Could you check a few things on this model? Use its own coordinates, in mm. A direction names the side the tool comes from. Give positions to 0.01 mm unless a question says otherwise; leave off trailing zeros. Write each loop counter-clockwise with the first axis right and the second up, starting at its lowest first coordinate (ties: lowest second). Pieces come first, ordered by that corner, then holes. Notation, with made-up numbers: (27.25, -21) -> (31.25, -21) arc R21 ccw to (31.25, 16) -> close; hole circle Ø10 at (-18, 85.5). An arc over 180 degrees is marked (long way). Write item = value, one per line. Start each with the question number.
Autodesk Inventor part; units mm, degrees
ref_plane "L_XY" through (12.2, 0, 0) normal (1, 0, 0) x (0, 0, -1)
ref_plane "L_YZ" through (12.2, 0, 0) normal (0, 0, -1) x (0, 1, 0)
ref_plane "L_ZX" through (12.2, 0, 0) normal (0, 1, 0) x (1, 0, 0)
sketch "Sketch_1" plane through (0, 0, 0) normal (0, 0, 1) x (1, 0, 0)
  line L0 (11.9, 0) -> (0, 0)
  line L1 (0, 0) -> (0, 8.2)
  line L2 (0, 8.2) -> (0.2, 8.4)
  line L3 (0.2, 8.4) -> (11.9, 8.4)
  line L4 (11.9, 8.4) -> (11.9, 0)
  line L5 (11.9, 0) -> (0, 0)
revolve "Revolution1" add sketch "Sketch_1" angle 360 about axis through (11.9, 0, 0) along (1, 0, 0)
sketch "Sketch_6" plane through (0, 0, 0) normal (1, 0, 0) x (0, 1, 0)
  line L0 (0, 0.6) -> (-8.4, 0.6)
  line L1 (-8.4, 0.6) -> (-8.4, -0.6)
  line L2 (-8.4, -0.6) -> (0, -0.6)
  line L3 (0, -0.6) -> (0, 0.6)
extrude "Extrusion1" cut sketch "Sketch_6" along normal blind 9
sketch "Sketch_7" plane through (4, 0, 0) normal (1, 0, 0) x (0, 0, -1)
  line L0 (-8.4, -5) -> (8.4, -5)
  line L1 (8.4, -5) -> (8.4, -7.75)
  line L2 (8.4, -7.75) -> (3, -7.75)
  line L3 (3, -7.75) -> (3, -6.5)
  line L4 (3, -6.5) -> (0.6, -6.5)
  line L5 (0.6, -6.5) -> (0.6, -5)
  line L6 (0.6, -5) -> (8.4, -5)
revolve "Revolution2" cut sketch "Sketch_7" angle 360 about axis through (4, -5, 8.4) along (0, 0, 1)
sketch "Sketch_13" plane through (4, 0, 0) normal (1, 0, 0) x (0, 0, -1)
  line L0 (-8.4, -5) -> (8.4, -5)
  line L1 (-0.6, -5) -> (-0.6, -6.2295)
  line L2 (-0.6, -6.2295) -> (-8.4, -6.2295)
  line L3 (-8.4, -6.2295) -> (-8.4, -5)
  line L4 (-8.4, -5) -> (-0.6, -5)
revolve "Revolution3" cut sketch "Sketch_13" angle 360 about axis through (4, -5, 8.4) along (0, 0, 1)
thread "Thread1"
sketch "Sketch_2" plane through (11.9, 0, 0) normal (1, 0, 0) x (0, 0, -1)
  line L0 (-9.4, 8.9) -> (-9.4, -8.9)
  line L1 (-9.4, -8.9) -> (9.4, -8.9)
  line L2 (9.4, -8.9) -> (9.4, 8.9)
  line L3 (9.4, 8.9) -> (-9.4, 8.9)
  line L4 (-8.4, 2.3) -> (-8.4, -2.3)
  line L5 (-8.4, -2.3) -> (8.4, -2.3)
  line L6 (8.4, -2.3) -> (8.4, 2.3)
  line L7 (8.4, 2.3) -> (-8.4, 2.3)
extrude "Extrusion2" cut sketch "Sketch_2" against normal blind 2.9
sketch "Sketch_3" plane through (0, 0, 0) normal (0, 0, 1) x (1, 0, 0)
  line L0 (11.9, 0) -> (0, 0)
  line L1 (0, 0) -> (0, 3)
  line L2 (0, 3) -> (11.9, 3)
  line L3 (11.9, 3) -> (11.9, 0)
  line L4 (11.9, 0) -> (0, 0)
revolve "Revolution4" cut sketch "Sketch_3" angle 360 about axis through (11.9, 0, 0) along (1, 0, 0)
sketch "Sketch_17" plane through (0, 0, 0) normal (1, 0, 0) x (0, 0, -1)
  line L0 (-0.6, 0) -> (0.6, 0)
  line L1 (0.6, 0) -> (0.6, 4.44)
  line L2 (0.6, 4.44) -> (-0.6, 4.44)
  line L3 (-0.6, 4.44) -> (-0.6, 0)
extrude "Extrusion3" cut sketch "Sketch_17" along normal blind 11.9
ref_plane "L_XY" through (12.2, 0, 0) normal (1, 0, 0) x (0, 0, -1)
ref_plane "L_YZ" through (12.2, 0, 0) normal (0, 0, -1) x (0, 1, 0)
ref_plane "L_ZX" through (12.2, 0, 0) normal (0, 1, 0) x (1, 0, 0)
ref_plane "screw_XY" through (4, -5, -3) normal (0, 0, -1) x (1, 0, 0)
ref_plane "screw_YZ" through (4, -5, -3) normal (1, 0, 0) x (0, -1, 0)
ref_plane "screw_ZX" through (4, -5, -3) normal (0, -1, 0) x (0, 0, -1)
properties part number "MCOC17-6_c"
(1) Imagine slicing it at C-C (x = 8.75). Please give me the cut outline in (y, z), then the cut area to 3 significant figures.
(2) We'd pull the mould along Z, two halves only. Please class faces 1 (the cylindrical face through (6, 0, 3)), 2 (the flat face through (9, -5, 4)): released by +Z, released by -Z, zero draft, split by the parting line, or undercut.
(3) Imagine slicing it at A-A (x = 10.75). Please give me the cut outline in (y, z).
(4) I'm going to push flat-ended pins straight in: pin 1 (1.5 mm diameter, centred on x = 10, z = 5, fed in from -Y); pin 2 (1.5 mm diameter, centred on x = 10, y = -2.5, fed in from +Z); pin 3 (6 mm diameter, centred on x = 9.5, y = -4.5, fed in from +Z) (3 decimals). Where does each tip first touch, or does it pass through?
(5) Imagine slicing it at D-D (x = 4). State how many separate pieces and enclosed holes the cut face has, then the cut area to 3 significant figures.
(6) Imagine slicing it at B-B (y = 0). Please give me the cut outline in (x, z).
(7) If I drill on line 1 along Y through (x, z) = (4, 2.5); line 2 along X through (y, z) = (-5, -2); line 3 along X through (y, z) = (-5, 3), over which ranges is the centre line in solid material (lowest first)? Write a range as from..to.
(8) On a 3-axis mill with a long thin cutter (end or side, diameter ignored), from which of +Z, -Z, +X, -X, +Y, -Y can I reach the whole of each face in a straight line? I mean faces 3 (the flat face through (4, 4, 0.6)), 4 (the cylindrical face through (6, 0, -3)), 5 (the cylindrical face through (5.265, -5.806, -1.783)), 6 (the flat face through (9, 5, 0)). Say none if no direction works.
Answers below:
q1.outline = (-8.38, -0.6) arc R8.4 ccw (long way) to (-8.38, 0.6) -> (-2.94, 0.6) arc R3 cw to (2.94, 0.6) -> (4.44, 0.6) -> (4.44, -0.6) -> (2.94, -0.6) arc R3 cw to (-2.94, -0.6) -> close
q1.area = 185 mm^2
q2.face_1 = undercut
q2.face_2 = zero draft
q3.outline = (-2.3, -8.08) arc R8.4 ccw to (2.3, -8.08) -> (2.3, -1.93) arc R3 cw to (-2.3, -1.93) -> close; (-2.3, 1.93) arc R3 cw to (2.3, 1.93) -> (2.3, 8.08) arc R8.4 ccw to (-2.3, 8.08) -> close
q4.pin_1 = -2.3
q4.pin_2 = 8.22
q4.pin_3 = 8.265
q5.separate_pieces = 3
q5.enclosed_holes = 0
q5.area = 144 mm^2
q6.outline = (0, -8.2) -> (0.2, -8.4) -> (11.9, -8.4) -> (11.9, -3) -> (0, -3) -> close; (0, 3) -> (11.9, 3) -> (11.9, 8.4) -> (0.2, 8.4) -> (0, 8.2) -> close
q7.line_1 = -8.02..-6.23, -3.77..-1.66, 1.66..8.02
q7.line_2 = 0..2.5, 5.5..9
q7.line_3 = 0..2.77, 5.23..9
q8.face_3 = +X, -X, -Y
q8.face_4 = +X, -X
q8.face_5 = -Z
q8.face_6 = +Z, -Z, +X, +Y
